from build123d import *

# Parameters (mm, degrees)
BOSS_EXTRUDE1_DEPTH             = 30
BOSS_EXTRUDE1_DEPTH_BACK        = 30
BOSS_EXTRUDE2_REACH             = 45.732
BOSS_EXTRUDE2_END_RADIUS        = 17.5
SKETCH3_R                       = 12
BOSS_EXTRUDE2_DIRECTION_2_DEPTH = 17
BOSS_EXTRUDE3_START             = 4
BOSS_EXTRUDE3_DEPTH             = 4
SKETCH5_W                       = 11
SKETCH5_H                       = 11
CUT_EXTRUDE1_DEPTH              = 17


with BuildPart() as part:
    # Sketch1 → Boss-Extrude1 (new, two sides: drawn at the far end of the back side and taken through both)
    with BuildSketch(Plane(origin=(0, 0, 0), x_dir=(0, 0, -1), z_dir=(1, 0, 0)).offset(-BOSS_EXTRUDE1_DEPTH_BACK)):
        with BuildLine():
            Line((-17.5, 0), (-22.5, 0))
            ThreePointArc((-22.5, 0), (0, -22.5), (22.5, 0))
            Line((22.5, 0), (17.5, 0))
            ThreePointArc((17.5, 0), (0, -17.5), (-17.5, 0))
        make_face()
    extrude(amount=BOSS_EXTRUDE1_DEPTH + BOSS_EXTRUDE1_DEPTH_BACK)

    # Boss-Extrude2: up to this cylinder (the profile starts inside it)
    boss_extrude2_end = Plane(origin=(0, 0, 0), z_dir=(1, 0, 0)) * Cylinder(BOSS_EXTRUDE2_END_RADIUS, 127.464, mode=Mode.PRIVATE)
    # Sketch3 → Boss-Extrude2 (add, up to the surface)
    with BuildSketch(Plane(origin=(0, 0, 0), x_dir=(1, 0, 0), z_dir=(0, 1, 0)), mode=Mode.PRIVATE) as boss_extrude2_sk1:
        with Locations(Location((0, 0, 0), (0, 0, 270))):
            Circle(SKETCH3_R)
    boss_extrude2_tool1 = extrude(boss_extrude2_sk1.sketch, amount=-BOSS_EXTRUDE2_REACH, mode=Mode.PRIVATE) & boss_extrude2_end
    add(boss_extrude2_tool1.solids().sort_by_distance((0, 0, 0))[0])

    # Sketch3 → Boss-Extrude2 direction 2 (add)
    with BuildSketch(Plane(origin=(0, 0, 0), x_dir=(1, 0, 0), z_dir=(0, 1, 0))):
        with Locations(Location((0, 0, 0), (0, 0, 270))):
            Circle(SKETCH3_R)
    extrude(amount=BOSS_EXTRUDE2_DIRECTION_2_DEPTH)

    # Sketch4 → Boss-Extrude3 (add)
    with BuildSketch(Plane.ZY.offset(30).offset(BOSS_EXTRUDE3_START)):
        with BuildLine():
            Line((-22.5, 0), (22.5, 0))
            ThreePointArc((22.5, 0), (0, -22.5), (-22.5, 0))
        make_face()
    extrude(amount=-BOSS_EXTRUDE3_DEPTH)

    # Sketch5 → Cut-Extrude1 (cut)
    with BuildSketch(Plane(origin=(0, 17, 0), x_dir=(1, 0, 0), z_dir=(0, 1, 0))):
        Rectangle(SKETCH5_W, SKETCH5_H)
    extrude(amount=-CUT_EXTRUDE1_DEPTH, mode=Mode.SUBTRACT)


solid = part.part
Could you check a few things on this model? Use its own coordinates, in mm. A direction names the side the tool comes from. Round coordinates to 2 decimals unless told otherwise and drop trailing zeros. Write each loop counter-clockwise with the first axis right and the second up, starting at its lowest first coordinate (ties: lowest second). Pieces come first, ordered by that corner, then holes. Notation, with made-up numbers: (60, 19) -> (99, 19) arc R19 ccw to (99, 31) -> close; hole circle Ø4 at (50.25, 25). An arc over 180 degrees is marked (long way). Use a Markdown table: item, result.
1. Please list where these lines run through material, in increasing order: probe 1 along Z at (x, y) = (8, -6.5); probe 2 along X at (y, z) = (6, 0.5); probe 3 along Z at (x, y) = (8, -10.5).
Answer key:
| item | result |
|---|---|
| probe 1 | z = -21.54 to -16.25, -8.94 to 8.94, 16.25 to 21.54 |
| probe 2 | x = -11.99 to -5.5, 5.5 to 11.99 |
| probe 3 | z = -19.9 to -14, -8.94 to 8.94, 14 to 19.9 |
2. If we section it at D-D (y = -19): List the corners of the cut face in (x, z) for me.
Answer key:
| item | result |
|---|---|
| outline | (-34, -12.05) -> (30, -12.05) -> (30, 12.05) -> (-34, 12.05) -> close |
3. We'd pull the mould along Z, two halves only. Please class faces 1 (the face through (-5.5, 9, 0)), 2 (the face through (30, -18, 0)), 3 (the face through (-2.448, -22.495, 0.495)), 4 (the face through (5.5, 9, 0)): +Z half, -Z half, draft (parallel to the pull), parting line (faces both ways), or undercut.
Answer key:
| item | result |
|---|---|
| face 1 | undercut |
| face 2 | draft |
| face 3 | parting line |
| face 4 | undercut |
4. For pin 1 Ø6 at (y, z) = (7, -16.5) entering from +X; pin 2 Ø3 at (y, z) = (-3.5, -9.5) entering from +X; pin 3 Ø8 at (x, z) = (19, -1) entering from +Y; pin 4 Ø3.5 at (y, z) = (10.5, -0.5) entering from -X, each with a flat end and sliding along its axis, tell me the tip position at first contact or that it passes through.
Answer key:
| item | result |
|---|---|
| pin 1 | passes through |
| pin 2 | stops at x = 8.94 |
| pin 3 | stops at y = -16.77 |
| pin 4 | stops at x = -12 |
5. If we section it at B-B (z = 0): List the corners of the cut face in (x, y) for me.
Answer key:
| item | result |
|---|---|
| outline | (-34, -22.5) -> (30, -22.5) -> (30, -17.5) -> (12, -17.5) -> (12, 17) -> (5.5, 17) -> (5.5, 0) -> (-5.5, 0) -> (-5.5, 17) -> (-12, 17) -> (-12, -17.5) -> (-30, -17.5) -> (-30, 0) -> (-34, 0) -> close |
6. If we section it at A-A (y = 13): List the corners of the cut face in (x, z) for me.
Answer key:
| item | result |
|---|---|
| outline | circle Ø24 at (0, 0); hole (-5.5, -5.5) -> (5.5, -5.5) -> (5.5, 5.5) -> (-5.5, 5.5) -> close |
7. If we section it at C-C (x = -4.5): List the corners of the cut face in (y, z) for me.
Answer key:
| item | result |
|---|---|
| outline | (-13.51, -11.12) -> (17, -11.12) -> (17, -5.5) -> (0, -5.5) -> (0, 5.5) -> (17, 5.5) -> (17, 11.12) -> (-13.51, 11.12) arc R17.5 cw to (0, 17.5) -> (0, 22.5) arc R22.5 ccw to (0, -22.5) -> (0, -17.5) arc R17.5 cw to start |
8. Which directions (+Z, -Z, +X, -X, +Y, -Y) give clear straight access to the entire face, cutting with the end or side of a thin tool? Please do faces 5 (the face through (-34, -9, 0)), 6 (the face through (3.604, -0.491, 11.446)), 7 (the face through (-9, 0, -18)).
Answer key:
| item | result |
|---|---|
| face 5 | +Z, -Z, -X, +Y, -Y |
| face 6 | +Y |
| face 7 | -X, +Y |
